Autodesk Inventor part; units mm, degrees
ref_plane "YZ Plane" through (0, 0, 0) normal (1, 0, 0) x (0, 1, 0)
ref_plane "XZ Plane" through (0, 0, 0) normal (0, 1, 0) x (-1, 0, 0)
ref_plane "XY Plane" through (0, 0, 0) normal (0, 0, 1) x (1, 0, 0)
sketch "スケッチ1" plane through (0, 0, 0) normal (0, 1, 0) x (-1, 0, 0)
  circle A0 centre (0, 0) radius 1.15
  circle A1 centre (0, 0) radius 2
  circle A2 centre (0, 0) radius 2.9
  line L0 (-2, 0) -> (2, 0)
  line L1 (2, 0) -> (2, -2.9)
  line L2 (2, -2.9) -> (-2, -2.9)
  line L3 (-2, -2.9) -> (-2, 0)
  line L4 (0, 0) -> (0, 2.9)
  line L5 (0, 0) -> (2.9, 0)
  line L6 (2.9, 0) -> (2.9, 15)
  line L7 (2.9, 15) -> (0, 15)
  line L8 (0, 15) -> (0, 0)
  line L9 (0, 0) -> (2.9, 0)
  line L10 (2.9, 0) -> (2.9, 10)
  line L11 (2.9, 10) -> (0, 10)
  line L12 (0, 10) -> (0, 0)
  point P0 (0, 2)
  point P1 (-2, -2.1)
  point P2 (2, -2.1)
  dimension "d1" = 4
  dimension "d2" = 5.8
  dimension "d0" = 2.3
  dimension "d3" = 15
  dimension "d4" = 10
extrude "押し出し1" add sketch "スケッチ1" along normal blind 3.3 contours A1 L3 A2 L4
extrude "押し出し2" add sketch "スケッチ1" along normal blind 4.5 contours L5 A2 L1 | A1 L4 A2 L5 | A2 L8 L11 L6
extrude "押し出し3" add sketch "スケッチ1" against normal blind 0.75 contours L0 A1 A0 | A0 L4 A1 L0 | A0 L0 A1 L4 | L1 A2 L3 A1 | L5 A2 L1 | A1 L4 A2 L5 | A1 L3 A2 L4 | A2 L8 L11 L6
sketch "スケッチ2" plane through (0, 4.5, 0) normal (0, 1, 0) x (1, 0, 0)
  circle A0 centre (0, 0) radius 1.15
  line L0 (-2, 0) -> (-2, 2.1)
  circle A1 centre (0, 0) radius 2
  arc A2 (-2, 2.1) -> (-2.9, 0) centre (0, 0) ccw
  circle A3 centre (0, 0) radius 2.9
  line L1 (-2, 0) -> (2, 0)
  line L2 (2, 0) -> (2, 2.9)
  line L3 (2, 2.9) -> (-2, 2.9)
  line L4 (-2, 2.9) -> (-2, 0)
  line L5 (-2.9, 0) -> (-2.9, -10)
  line L6 (-2.9, -10) -> (0, -10)
  line L7 (-2.9, 0) -> (0, 0)
  line L8 (0, 0) -> (0, -10)
  line L9 (0, -10) -> (-2.9, -10)
  line L10 (-2.9, -10) -> (-2.9, 0)
  point P0 (0, -2.9)
extrude "押し出し4" add sketch "スケッチ2" along normal blind 0.75 contours L1 A1 L8 A0 | A0 L1 A1 | A0 L8 A1 L1 | L2 A3 L8 A1 | A1 L0 A3 L2 | L7 A2 L0 | A1 L8 A3 L7 | A3 L8 L6 L5
sketch "スケッチ3" plane through (-2.9, -0.75, 10) normal (0, 0, 1) x (1, 0, 0)
  line L0 (4.05, 0) -> (1.75, 0)
  line L1 (0, 0) -> (0, 6)
  line L2 (2.9, 0) -> (0, 0)
  line L3 (0, 0) -> (0, 0.75)
  line L4 (0, 0.75) -> (2.9, 0.75)
  line L5 (2.9, 0.75) -> (2.9, 0)
  line L6 (2.9, 0.75) -> (1.4, 0.75)
  line L7 (1.4, 0.75) -> (1.4, 1.15)
  line L8 (1.4, 1.15) -> (2.9, 1.15)
  line L9 (2.9, 1.15) -> (2.9, 0.75)
  line L10 (1.4, 0.75) -> (1.4, 1.25)
  dimension "d13" = 1.5
  dimension "d14" = 0.4
  dimension "d15" = 0.5
hole "穴1" at (-1.5, 0.5, 10) direction (0, 0, -1) diameter 1 end through all
sketch "スケッチ4" plane through (-2.9, -0.75, 10) normal (0, 0, 1) x (1, 0, 0)
  line L0 (0, 0) -> (0, 6)
  line L1 (0, 6) -> (4, 6)
  line L2 (4, 6) -> (4, 2)
  line L3 (4, 2) -> (0, 2)
  line L4 (0, 2) -> (0, 6)
  point P0 (2.9, 0.75)
  dimension "d23" = 4
  dimension "d24" = 4
extrude "押し出し5" add sketch "スケッチ4" along normal blind 8 and the other way blind 3
sketch "スケッチ5" plane through (-2.9, -0.75, 18) normal (0, 0, 1) x (1, 0, 0)
  line L0 (5.8, 6) -> (0, 6)
  line L1 (0, 6) -> (2, 6)
  line L2 (2, 6) -> (2, 4)
  line L3 (2, 4) -> (0, 4)
  line L4 (0, 4) -> (0, 6)
  point P0 (2.9, 0.75)
  point P1 (2.9, 6)
  dimension "d29" = 2
  dimension "d30" = 2
hole "穴2" at (-0.9, 3.25, 18) direction (0, 0, -1) diameter 2.3 depth 10
fillet "フィレット1" radius 2 1 edges at (1.1, 3.25, 7)
properties part number "srod1.3"
Here's how the part is built. I have some questions about the finished solid (model axes, mm). A direction names the side the tool comes from. Give positions to 0.01 mm unless a question says otherwise; leave off trailing zeros. Order: outer loops, then holes, each group sorted by start corner. A loop starts at its lowest first (then second) coordinate and runs counter-clockwise, first axis right, second up. Notation, with made-up numbers: M 22.5,3.25 L 30.5,3.25 A27 cw 30.5,32.25 Z; hole C 37,70 d9. An arc over 180 degrees is marked long. Answer as a JSON object with one key per item and string values. Group by question number.
1) Suppose I cut it at D-D, the plane z = -0.5. Write out the boundary of the cut face in (x, y).
2) Please list where these lines run through material, in increasing order: L1, parallel to Y at x = -0.9, z = 13.25; L2, parallel to Y at x = -1.5, z = 4.5; L3, parallel to X at y = -0.25, z = 0. Write a range as [from, to].
3) I'm going to push flat-ended pins straight in: pin 1 Ø2 at (y, z) = (3.5, 14.5) entering from +X; pin 2 Ø2 at (x, y) = (-0.9, 3.25) entering from +Z; pin 3 Ø2.5 at (y, z) = (2, -1.5) entering from -X. Where does each tip first touch, or does it pass through?
4) Suppose I cut it at B-B, the plane x = 2.3. Write out the boundary of the cut face in (y, z), plus the area to 3 significant figures.
5) Suppose I cut it at A-A, the plane z = 15.5. Write out the boundary of the cut face in (x, y).
6) Suppose I cut it at C-C, the plane y = -0.25. Write out the boundary of the cut face in (x, z).
7) On a 3-axis mill with a long thin cutter (end or side, diameter ignored), from which of +Z, -Z, +X, -X, +Y, -Y can I reach the whole of each face in a straight line? I mean faces 4 (the flat face through (1, 4.5, -1)), 5 (the cylindrical face through (0.81, 3.28, 7.75)), 6 (the cylindrical face through (-0.46, 2.188, 12.93)), 7 (the flat face through (2, 2, -1)). Say none if no direction works.
8) We'd pull the mould along Z, two halves only. Please class faces 1 (the flat face through (0, 0, -2)), 2 (the cylindrical face through (-0.91, 4.87, -0.7)), 3 (the flat face through (-1, 3, 8)): pulls with the +Z half, pulls with the -Z half, needs draft (parallel to the pull), parting line crosses it, or undercut.
Results found:
{
 "1": {"outline": "M -2.86,-0.75 L -1.04,-0.75 L -1.04,0 L -2,0 L -2,4.5 L -1.04,4.5 L -1.04,5.25 L -2.86,5.25 Z; M 1.04,-0.75 L 2.86,-0.75 L 2.86,3.3 L 2,3.3 L 2,0 L 1.04,0 Z; M 1.04,4.5 L 2.86,4.5 L 2.86,5.25 L 1.04,5.25 Z"},
 "2": {"L1": "[1.25, 2.1], [4.4, 5.25]", "L2": "[-0.75, 0], [1, 5.25]", "L3": "[-2.9, -1.15], [1.15, 2.9]"},
 "3": {"pin 1": "x = 1.1", "pin 2": "z = 8", "pin 3": "x = -2.89"},
 "4": {"outline": "M -0.75,-1.77 L 3.3,-1.77 L 3.3,1.77 L -0.75,1.77 Z; M 4.5,-1.77 L 5.25,-1.77 L 5.25,1.77 L 4.5,1.77 Z", "area": "17.0 mm²"},
 "5": {"outline": "M -2.9,1.25 L 1.1,1.25 L 1.1,5.25 L -2.9,5.25 Z; hole C -0.9,3.25 d2.3"},
 "6": {"outline": "M -2.9,0 A2.9 ccw long 0,2.9 L 0,10 L -2.9,10 Z; hole C 0,0 d2.3"},
 "7": {"face 4": "-Z, +X", "face 5": "+X, +Y, -Y", "face 6": "+Z", "face 7": "-Z"},
 "8": {"face 1": "needs draft", "face 2": "undercut", "face 3": "pulls with the +Z half"}
}
